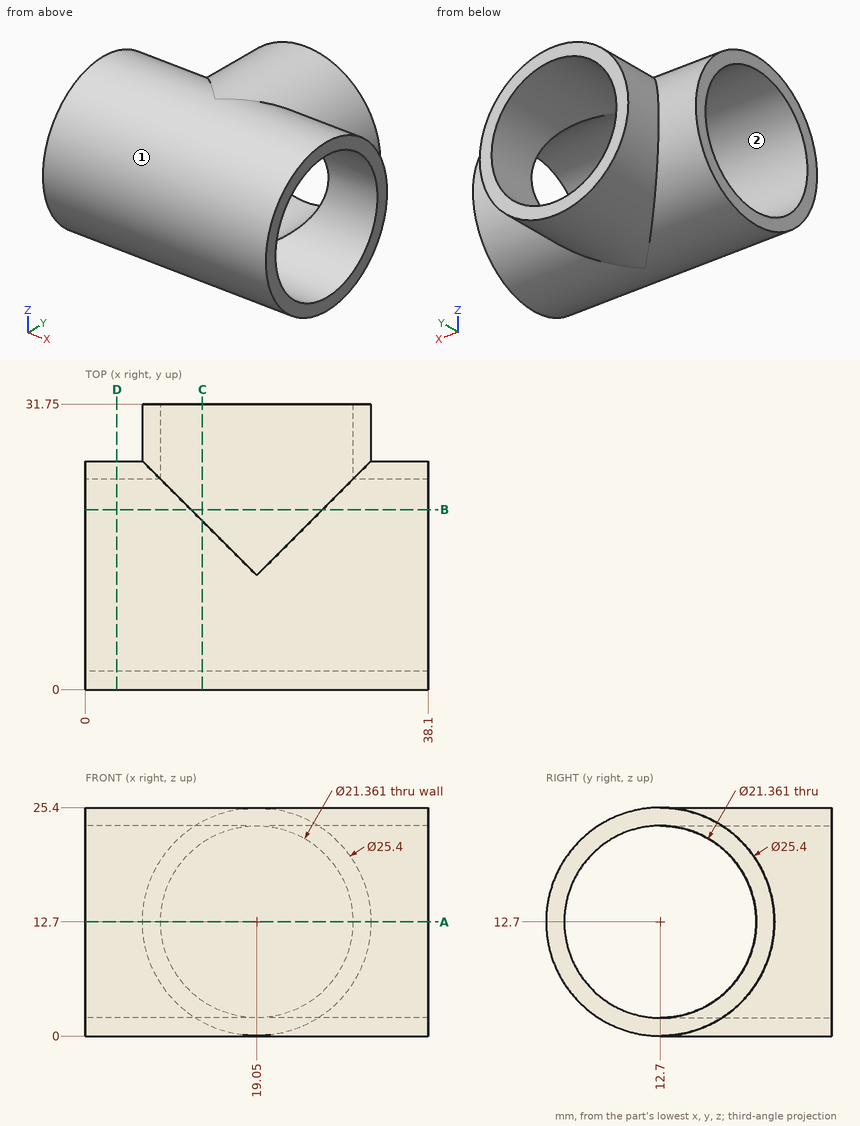
Job drawing, mm, ordinate dimensions from the low corner. One solid piece. Round coordinates to 2 decimals unless told otherwise and drop trailing zeros. Loops run counter-clockwise (first coordinate to the right, second up) from the corner with the lowest first, then second, coordinate; pieces in that order, holes last. Notation, with made-up numbers: (-12, 56.25) -> (34, 56.25) arc R23 cw to (34, 81.25) -> close; hole circle Ø11 at (43.5, 64.25). An arc over 180 degrees is marked (long way). One line per item, written item: value. Start each with the question number.
Q1. Cut at C-C on x = 13. List the corners of the cut face in (y, z).
Q2. Two-plate mould, pull along Y, no slides. Class the marked faces 1 and 2: released by +Y, released by -Y, zero draft, split by the parting line, or undercut.
Q3. Drop flat-ended pins along their axis: pin 1 Ø2 at (x, z) = (14.5, 19) entering from +Y; pin 2 Ø6 at (x, z) = (12.5, 18) entering from -Y; pin 3 Ø1.5 at (x, y) = (16.5, 8) entering from +Z. Give the stop position or say it passes through.
Q4. Cut at D-D on x = 3.5. List the corners of the cut face in (y, z).
Q5. Cut at B-B on y = 20. List the corners of the cut face in (x, z).
Q6. Cut at A-A on z = 12.7. List the corners of the cut face in (x, y).
Q7. Probe line 1 along Z through (x, y) = (21, 12.7); line 2 along X through (y, z) = (24.25, 12.7); line 3 along X through (y, z) = (27.25, 12.7). List the from-to ranges inside material, lowest first.
Computed:
1. outline: (18.75, 1.53) -> (31.75, 1.53) -> (31.75, 3.9) -> (18.75, 3.9) arc R10.68 cw (long way) to (18.75, 21.5) -> (31.75, 21.5) -> (31.75, 23.87) -> (18.75, 23.87) arc R12.7 ccw (long way) to start
2. face 1: split by the parting line
2. face 2: undercut
3. pin 1: y = 4.9
3. pin 2: y = 0.21
3. pin 3: z = 24.77
4. outline: circle Ø25.4 at (12.7, 12.7); hole circle Ø21.36 at (12.7, 12.7)
5. outline: (0, 2.31) -> (11.75, 2.31) arc R12.7 ccw to (26.35, 2.31) -> (38.1, 2.31) -> (38.1, 4.9) -> (26.35, 4.9) arc R10.68 cw to (11.75, 4.9) -> (0, 4.9) -> close; (0, 20.5) -> (11.75, 20.5) arc R10.68 cw to (26.35, 20.5) -> (38.1, 20.5) -> (38.1, 23.09) -> (26.35, 23.09) arc R12.7 ccw to (11.75, 23.09) -> (0, 23.09) -> close
6. outline: (0, 0) -> (38.1, 0) -> (38.1, 2.02) -> (0, 2.02) -> close; (0, 23.38) -> (8.37, 23.38) -> (8.37, 31.75) -> (6.35, 31.75) -> (6.35, 25.4) -> (0, 25.4) -> close; (29.73, 23.38) -> (38.1, 23.38) -> (38.1, 25.4) -> (31.75, 25.4) -> (31.75, 31.75) -> (29.73, 31.75) -> close
7. line 1: 0 to 2.02, 23.38 to 25.4
7. line 2: 0 to 8.37, 29.73 to 38.1
7. line 3: 6.35 to 8.37, 29.73 to 31.75
